from build123d import *

# Parameters (mm, degrees)
SKETCH1_R           = 1.25
SKETCH1_R_2         = 16.5
BOSS_EXTRUDE1_DEPTH = 3.15
SKETCH2_W           = 42
SKETCH2_H           = 34
BOSS_EXTRUDE2_DEPTH = 3.15
FILLET1_R           = 50
SKETCH3_W           = 20
SKETCH3_H           = 3.16
CUT_EXTRUDE1_DEPTH  = 255.013877696
SKETCH4_R           = 1.4
CUT_EXTRUDE2_DEPTH  = 10
SKETCH5_R           = 1.4
CUT_EXTRUDE3_DEPTH  = 10
CUT_EXTRUDE4_DEPTH  = 255.013877696
SKETCH8_W           = 218.2
SKETCH8_H           = 1.5
BOSS_EXTRUDE3_DEPTH = 3.15


with BuildPart() as part:
    # Sketch1 → Boss-Extrude1 (new body)
    with BuildSketch(Plane(origin=(0, 11.030201327, 0), x_dir=(1, 0, 0), z_dir=(0, 1, 0))):
        Polygon((-162.156726515, -108.167379901), (-194.899872265, -108.167379901), (-199.52829939, -108.167379901), (-199.52829939, 34.111047224), (-199.52829939, 66.854192974), (-199.52829939, 71.482620099), (-194.899872265, 71.482620099), (-162.156726515, 71.482620099), (-157.52829939, 71.482620099), (-157.52829939, -108.167379901), align=None)
        with Locations(Location((-163.02829939, 65.982620099, 0), (0, 0, 270))):
            Circle(SKETCH1_R, mode=Mode.SUBTRACT)
        with Locations(Location((-163.02829939, 34.982620099, 0), (0, 0, 270))):
            Circle(SKETCH1_R, mode=Mode.SUBTRACT)
        with Locations(Location((-194.02829939, 34.982620099, 0), (0, 0, 270))):
            Circle(SKETCH1_R, mode=Mode.SUBTRACT)
        with Locations(Location((-194.02829939, 65.982620099, 0), (0, 0, 270))):
            Circle(SKETCH1_R, mode=Mode.SUBTRACT)
        with Locations(Location((-163.02829939, -102.667379901, 0), (0, 0, 270))):
            Circle(SKETCH1_R, mode=Mode.SUBTRACT)
        with Locations(Location((-163.02829939, -71.667379901, 0), (0, 0, 270))):
            Circle(SKETCH1_R, mode=Mode.SUBTRACT)
        with Locations(Location((-194.02829939, -102.667379901, 0), (0, 0, 270))):
            Circle(SKETCH1_R, mode=Mode.SUBTRACT)
        with Locations(Location((-194.02829939, -71.667379901, 0), (0, 0, 270))):
            Circle(SKETCH1_R, mode=Mode.SUBTRACT)
        with Locations(Location((-178.52829939, -87.167379901, 0), (0, 0, 270))):
            Circle(SKETCH1_R_2, mode=Mode.SUBTRACT)
        with Locations(Location((-178.52829939, 50.482620099, 0), (0, 0, 270))):
            Circle(SKETCH1_R_2, mode=Mode.SUBTRACT)
    extrude(amount=BOSS_EXTRUDE1_DEPTH)

    # Sketch2 → Boss-Extrude2 (add)
    with BuildSketch(Plane(origin=(0, 14.180201327, 0), x_dir=(1, 0, 0), z_dir=(0, 1, 0))):
        Polygon((-157.52829939, -144.167379901), (-157.52829939, -142.167379901), (-157.52829939, -108.167379901), (-199.52829939, -108.167379901), (-199.52829939, -142.167379901), (-199.52829939, -157.167379901), (-157.52829939, -157.167379901), (60.67170061, -157.167379901), (60.67170061, -144.167379901), (45.67170061, -144.167379901), align=None)
        with Locations((-178.52829939, 88.482620099)):
            Rectangle(SKETCH2_W, SKETCH2_H)
        Polygon((-199.52829939, 105.482620099), (-157.52829939, 105.482620099), (-157.52829939, 107.482620099), (45.67170061, 107.482620099), (60.67170061, 107.482620099), (60.67170061, 120.482620099), (-157.52829939, 120.482620099), (-199.52829939, 120.482620099), align=None)
    extrude(amount=-BOSS_EXTRUDE2_DEPTH)

    # Fillet1
    fillet1_edges = [part.edges().sort_by_distance(p)[0] for p in [
        (-199.52829939, 12.605201327, 157.167379901),
        (-199.52829939, 12.605201327, -120.482620099),
    ]]
    fillet(fillet1_edges, radius=FILLET1_R)

    # Sketch3 → Cut-Extrude1 (cut, through all)
    with BuildSketch(Plane(origin=(0, 14.180201327, 0), x_dir=(1, 0, 0), z_dir=(0, 1, 0))):
        with Locations((-94.42829939, 118.902620099)):
            Rectangle(SKETCH3_W, SKETCH3_H)
        with Locations((-134.42829939, 118.902620099)):
            Rectangle(SKETCH3_W, SKETCH3_H)
        with Locations((-54.42829939, 118.902620099)):
            Rectangle(SKETCH3_W, SKETCH3_H)
        with Locations((-14.42829939, 118.902620099)):
            Rectangle(SKETCH3_W, SKETCH3_H)
        with Locations((25.57170061, 118.902620099)):
            Rectangle(SKETCH3_W, SKETCH3_H)
        with Locations((25.57170061, -155.587379901)):
            Rectangle(SKETCH3_W, SKETCH3_H)
        with Locations((-14.42829939, -155.587379901)):
            Rectangle(SKETCH3_W, SKETCH3_H)
        with Locations((-54.42829939, -155.587379901)):
            Rectangle(SKETCH3_W, SKETCH3_H)
        with Locations((-94.42829939, -155.587379901)):
            Rectangle(SKETCH3_W, SKETCH3_H)
        with Locations((-134.42829939, -155.587379901)):
            Rectangle(SKETCH3_W, SKETCH3_H)
    extrude(amount=-CUT_EXTRUDE1_DEPTH, mode=Mode.SUBTRACT)

    # Sketch4 → Cut-Extrude2 (cut)
    with BuildSketch(Plane(origin=(0, 14.180201327, 0), x_dir=(1, 0, 0), z_dir=(0, 1, 0))):
        with Locations(Location((-177.812570637, 98.766891346, 0), (0, 0, 270))):
            Circle(SKETCH4_R)
        with Locations(Location((-177.812570637, -135.451651148, 0), (0, 0, 270))):
            Circle(SKETCH4_R)
    extrude(amount=-CUT_EXTRUDE2_DEPTH, mode=Mode.SUBTRACT)

    # Sketch5 → Cut-Extrude3 (cut)
    with BuildSketch(Plane(origin=(0, 14.180201327, 0), x_dir=(1, 0, 0), z_dir=(0, 1, 0))):
        with Locations(Location((53.12170061, 111.647620099, 0), (0, 0, 270))):
            Circle(SKETCH5_R)
        with Locations(Location((53.12170061, -148.342379901, 0), (0, 0, 270))):
            Circle(SKETCH5_R)
        with Locations(Location((23.12170061, 111.647620099, 0), (0, 0, 270))):
            Circle(SKETCH5_R)
        with Locations(Location((23.12170061, -148.342379901, 0), (0, 0, 270))):
            Circle(SKETCH5_R)
    extrude(amount=-CUT_EXTRUDE3_DEPTH, mode=Mode.SUBTRACT)

    # Sketch6 → Cut-Extrude4 (cut, through all)
    with BuildSketch(Plane(origin=(0, 14.180201327, 0), x_dir=(1, 0, 0), z_dir=(0, 1, 0))):
        with BuildLine():
            Line((-161.77829939, 69.982620099), (-161.77829939, 65.982620099))
            ThreePointArc((-161.77829939, 65.982620099), (-163.02829939, 64.732620099), (-164.27829939, 65.982620099))
            Line((-164.27829939, 65.982620099), (-164.27829939, 69.982620099))
            ThreePointArc((-164.27829939, 69.982620099), (-163.02829939, 71.232620099), (-161.77829939, 69.982620099))
        make_face()
        with BuildLine():
            Line((-161.77829939, 38.982620099), (-161.77829939, 34.982620099))
            ThreePointArc((-161.77829939, 34.982620099), (-163.02829939, 33.732620099), (-164.27829939, 34.982620099))
            Line((-164.27829939, 34.982620099), (-164.27829939, 38.982620099))
            ThreePointArc((-164.27829939, 38.982620099), (-163.02829939, 40.232620099), (-161.77829939, 38.982620099))
        make_face()
        with BuildLine():
            Line((-192.77829939, 38.982620099), (-192.77829939, 34.982620099))
            ThreePointArc((-192.77829939, 34.982620099), (-194.02829939, 33.732620099), (-195.27829939, 34.982620099))
            Line((-195.27829939, 34.982620099), (-195.27829939, 38.982620099))
            ThreePointArc((-195.27829939, 38.982620099), (-194.02829939, 40.232620099), (-192.77829939, 38.982620099))
        make_face()
        with BuildLine():
            Line((-195.27829939, 69.982620099), (-195.27829939, 65.982620099))
            ThreePointArc((-195.27829939, 65.982620099), (-194.02829939, 64.732620099), (-192.77829939, 65.982620099))
            Line((-192.77829939, 65.982620099), (-192.77829939, 69.982620099))
            ThreePointArc((-192.77829939, 69.982620099), (-194.02829939, 71.232620099), (-195.27829939, 69.982620099))
        make_face()
        with BuildLine():
            Line((-162.02829939, 54.482620099), (-162.02829939, 50.482620099))
            ThreePointArc((-162.02829939, 50.482620099), (-178.52829939, 33.982620099), (-195.02829939, 50.482620099))
            Line((-195.02829939, 50.482620099), (-195.02829939, 54.482620099))
            ThreePointArc((-195.02829939, 54.482620099), (-178.52829939, 70.982620099), (-162.02829939, 54.482620099))
        make_face()
        with BuildLine():
            Line((-195.02829939, -91.167379901), (-195.02829939, -87.167379901))
            ThreePointArc((-195.02829939, -87.167379901), (-178.52829939, -70.667379901), (-162.02829939, -87.167379901))
            Line((-162.02829939, -87.167379901), (-162.02829939, -91.167379901))
            ThreePointArc((-162.02829939, -91.167379901), (-178.52829939, -107.667379901), (-195.02829939, -91.167379901))
        make_face()
        with BuildLine():
            Line((-192.77829939, -106.667379901), (-192.77829939, -102.667379901))
            ThreePointArc((-192.77829939, -102.667379901), (-194.02829939, -101.417379901), (-195.27829939, -102.667379901))
            Line((-195.27829939, -102.667379901), (-195.27829939, -106.667379901))
            ThreePointArc((-195.27829939, -106.667379901), (-194.02829939, -107.917379901), (-192.77829939, -106.667379901))
        make_face()
        with BuildLine():
            Line((-195.27829939, -71.667379901), (-195.27829939, -75.667379901))
            ThreePointArc((-195.27829939, -75.667379901), (-194.02829939, -76.917379901), (-192.77829939, -75.667379901))
            Line((-192.77829939, -75.667379901), (-192.77829939, -71.667379901))
            ThreePointArc((-192.77829939, -71.667379901), (-194.02829939, -70.417379901), (-195.27829939, -71.667379901))
        make_face()
        with BuildLine():
            Line((-164.27829939, -71.667379901), (-164.27829939, -75.667379901))
            ThreePointArc((-164.27829939, -75.667379901), (-163.02829939, -76.917379901), (-161.77829939, -75.667379901))
            Line((-161.77829939, -75.667379901), (-161.77829939, -71.667379901))
            ThreePointArc((-161.77829939, -71.667379901), (-163.02829939, -70.417379901), (-164.27829939, -71.667379901))
        make_face()
        with BuildLine():
            Line((-164.27829939, -102.667379901), (-164.27829939, -106.667379901))
            ThreePointArc((-164.27829939, -106.667379901), (-163.02829939, -107.917379901), (-161.77829939, -106.667379901))
            Line((-161.77829939, -106.667379901), (-161.77829939, -102.667379901))
            ThreePointArc((-161.77829939, -102.667379901), (-163.02829939, -101.417379901), (-164.27829939, -102.667379901))
        make_face()
    extrude(amount=-CUT_EXTRUDE4_DEPTH, mode=Mode.SUBTRACT)

    # Sketch8 → Boss-Extrude3 (add)
    with BuildSketch(Plane(origin=(0, 14.180201327, 0), x_dir=(1, 0, 0), z_dir=(0, 1, 0))):
        with Locations((-48.42829939, -143.417379901)):
            Rectangle(SKETCH8_W, SKETCH8_H)
        with Locations((-48.42829939, 106.732620099)):
            Rectangle(SKETCH8_W, SKETCH8_H)
    extrude(amount=-BOSS_EXTRUDE3_DEPTH)


solid = part.part
The model under review builds one solid part; all positions refer to its coordinate system, in mm. A direction names the side the tool comes from. Round coordinates to 2 decimals unless told otherwise and drop trailing zeros. Order: outer loops, then holes, each group sorted by start corner. A loop starts at its lowest first (then second) coordinate and runs counter-clockwise, first axis right, second up. Notation, with made-up numbers: (0.25, 48) -> (13.25, 48) arc R16 ccw to (13.25, 53) -> close; hole circle Ø3 at (-21, 84). An arc over 180 degrees is marked (long way). Write item = value, one per line. Start each with the question number.
Item 1: For faces 1 (the face through (-178.891, 12.583, -33.987)), 2 (the face through (-184.5, 12.6, 142.9)), list the 3-axis set-ups (+Z, -Z, +X, -X, +Y, -Y) from which the entire face can be reached by the end or side of a thin tool; tool diameter is ignored.
Item 2: Clearance check with flat-ended pins moving along their axes: pin 1 Ø1.6 at (x, y) = (-23.5, 12.5) entering from +Z; pin 2 Ø1.6 at (y, z) = (12, -68.5) entering from +X; pin 3 Ø0.9 at (x, y) = (-99, 13) entering from -Z. State where each tip first meets the part, or that it passes through.
Item 3: For line 1 along Z through (x, y) = (-52.5, 11.65); line 2 along Z through (x, y) = (-84, 11.75); line 3 along X through (y, z) = (11.85, -52.5), list the stretches that pass through material, from the lowest coordinate up.
Item 4: Consider section A-A on x = -18.5. Write out the cut boundary in (y, z), plus the area to 3 significant figures.
Item 5: Consider section C-C on y = 11.75. Count the separate pieces of the cut face and the enclosed holes in it, plus the area to 3 significant figures.
Item 6: Consider section D-D on z = -17.5. Write out the cut boundary in (x, y).
Item 7: Consider section B-B on x = 42.5. Write out the cut boundary in (y, z), plus the area to 4 significant figures.
Item 8: Mouldability with a two-part tool opening along Z and no side actions: class faces 3 (the face through (-178.89, 12.63, -70.98)), 4 (the face through (-166, 11.03, 18)), 5 (the face through (-185.27, 12.58, -105.45)) as released by +Z, released by -Z, zero draft, split by the parting line, or undercut.
Conclusion:
q1.face_1 = +Y, -Y
q1.face_2 = +Z, -X, +Y, -Y
q2.pin_1 = 154.01
q2.pin_2 = -157.53
q2.pin_3 = -117.32
q3.line_1 = -117.32 to -105.98, 142.67 to 154.01
q3.line_2 = -120.48 to -105.98, 142.67 to 157.17
q3.line_3 = -199.53 to -195.03, -162.03 to -157.53
q4.outline = (11.03, -117.32) -> (14.18, -117.32) -> (14.18, -105.98) -> (11.03, -105.98) -> close; (11.03, 142.67) -> (14.18, 142.67) -> (14.18, 154.01) -> (11.03, 154.01) -> close
q4.area = 71.4 mm2
q5.separate_pieces = 1
q5.enclosed_holes = 16
q5.area = 14,200 mm2
q6.outline = (-199.53, 11.03) -> (-157.53, 11.03) -> (-157.53, 14.18) -> (-199.53, 14.18) -> close
q7.outline = (11.03, -120.48) -> (14.18, -120.48) -> (14.18, -105.98) -> (11.03, -105.98) -> close; (11.03, 142.67) -> (14.18, 142.67) -> (14.18, 157.17) -> (11.03, 157.17) -> close
q7.area = 91.35 mm2
q8.face_3 = undercut
q8.face_4 = zero draft
q8.face_5 = released by -Z
